CAD build for the part. Positions are in the model's coordinates, mm. Face numbers are marked on the shaded views. A direction names the side the tool comes from. Coordinates: 2 decimals unless noted, no trailing zeros. Write each loop counter-clockwise with the first axis right and the second up, starting at its lowest first coordinate (ties: lowest second). Pieces come first, ordered by that corner, then holes. Notation, with made-up numbers: (14, -13) - (49, -13) arc R26 ccw to (49, 1) - close; hole circle Ø1 at (46.25, -13). An arc over 180 degrees is marked (long way). Answer in a Markdown table with one row per item. Add a question column.
Q1. Band-saw the part on A-A (y = -3). List the corners of the cut face in (x, z).
Q2. Band-saw the part on C-C (z = -48). List the corners of the cut face in (x, y), and give its area (3 significant figures).
Q3. Pin check, flat tips, straight feed: pin 1 (2 mm diameter, centred on x = -77, z = -52.5, fed in from -Y); pin 2 (1.5 mm diameter, centred on x = -53, y = -4.5, fed in from +Z); pin 3 (8 mm diameter, centred on x = 34.5, y = -19, fed in from +Z). Stop position of each tip, or through.
Q4. Two-plate mould, pull along X, no slides. Class the marked faces 1, 2 and 3: +X half, -X half, draft (parallel to the pull), parting line (faces both ways), or undercut.
Q5. 3-axis set-ups, long thin cutter, end or side, ignore diameter. For the marked faces 4, 5, 6 and 7: which of +Z, -Z, +X, -X, +Y, -Y reach the whole face in a straight line?
Q6. Band-saw the part on B-B (x = 40). List the corners of the cut face in (y, z).
Q7. Band-saw the part on D-D (x = -35). List the corners of the cut face in (y, z).
Q8. Drill centre lines: line 1 along X through (y, z) = (-7, -26); line 2 along X through (y, z) = (-7, -30); line 3 along Z through (x, y) = (31.5, -21.5). Where is each one in solid material? Low to high. Write a range as from..to.
```python
from build123d import *

# Parameters (mm, degrees)
F0_W      = 160
F0_H      = 100
F1_DEPTH  = 20
F3_W      = 27
F3_H      = 100
F4_DEPTH  = 20
F5_DEPTH  = 20
F6_R      = 10
F7_DEPTH  = 30
F9_W      = 160
F9_H      = 27
F10_DEPTH = 20
F11_DEPTH = 20
F12_DEPTH = 20
F13_DEPTH = 20


with BuildPart() as f1:
    # F0 (on Front) → F1 (new body)
    with BuildSketch(Plane.XZ):
        Rectangle(F0_W, F0_H)
    extrude(amount=-F1_DEPTH)

    # F3 (on offset) → F4 (join)
    with BuildSketch(Plane.YZ.offset(-80)):
        with Locations((-13.5, 0)):
            Rectangle(F3_W, F3_H)
    extrude(amount=-F4_DEPTH)

    # F5 (add): faces of the model
    f5_faces = [f1.faces().sort_by_distance(p)[0] for p in [
        (-90, -27, 0),
        (-90, 0, 0),
    ]]
    extrude(f5_faces, amount=-F5_DEPTH, dir=(0, -1, 0))

    # F6 (on face) → F7 (join)
    with BuildSketch(Plane.XZ):
        with Locations((-40, -26.8495120108)):
            Circle(F6_R)
        with Locations((-40, 23.1504879892)):
            Circle(F6_R)
        with Locations((40, -26.8495120108)):
            Circle(F6_R)
        with Locations((40, 23.1504879892)):
            Circle(F6_R)
    extrude(amount=F7_DEPTH)



with BuildPart() as f10:
    # F9 (on offset) → F10 (new body)
    with BuildSketch(Plane.XY.offset(-50)):
        with Locations((0, -13.5)):
            Rectangle(F9_W, F9_H)
    extrude(amount=-F10_DEPTH)


with BuildPart() as f11:
    # F11 (new, through all): a face of the model
    f11_faces = [f10.part.faces().sort_by_distance(p)[0] for p in [
        (0, 0, -60),
    ]]
    extrude(f11_faces, amount=F11_DEPTH)


with BuildPart() as f12:
    # F12 (new, through all): a face of the model
    f12_faces = [f10.part.faces().sort_by_distance(p)[0] for p in [
        (-80, -13.5, -60),
    ]]
    extrude(f12_faces, amount=F12_DEPTH)


with BuildPart() as f1_1:
    add(f1.part)
    # F13 (add, through all): a face of the model
    f13_faces = [f11.part.faces().sort_by_distance(p)[0] for p in [
        (-80, 10, -60),
    ]]

    add(f10.part)  # F13 merges F10

    add(f11.part)  # F13 merges F11

    add(f12.part)  # F13 merges F12
    extrude(f13_faces, amount=F13_DEPTH)


solid = f1_1.part
```
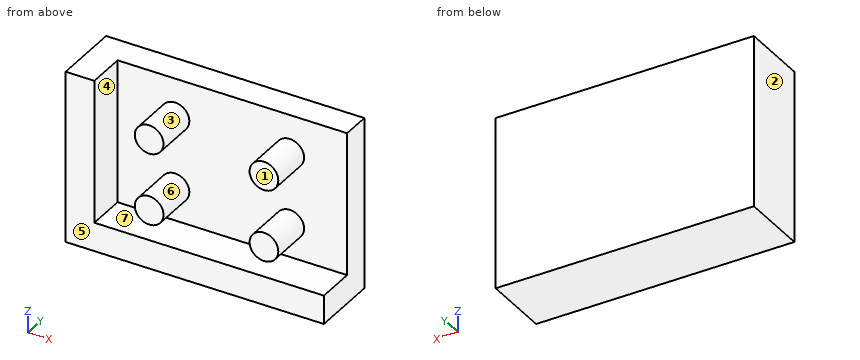
Checked values:
| question | item | result |
|---|---|---|
| 1 | outline | (-100, -70) - (80, -70) - (80, -50) - (-80, -50) - (-80, 50) - (-100, 50) - close; circle Ø20 at (-40, -26.85); circle Ø20 at (-40, 23.15); circle Ø20 at (40, -26.85); circle Ø20 at (40, 23.15) |
| 2 | outline | (-100, -27) - (-80, -27) - (-80, 0) - (80, 0) - (80, 20) - (-100, 20) - close |
| 2 | area | 4,140 mm² |
| 3 | pin 1 | stops at y = -27 |
| 3 | pin 2 | stops at z = -50 |
| 3 | pin 3 | stops at z = 33.04 |
| 4 | face 1 | draft |
| 4 | face 2 | -X half |
| 4 | face 3 | undercut |
| 5 | face 4 | +Z, -Y |
| 5 | face 5 | -Z, -X, -Y |
| 5 | face 6 | -Y |
| 5 | face 7 | +X, -Y |
| 6 | outline | (-30, -36.85) - (0, -36.85) - (0, -50) - (-27, -50) - (-27, -70) - (20, -70) - (20, 50) - (0, 50) - (0, 33.15) - (-30, 33.15) - (-30, 13.15) - (0, 13.15) - (0, -16.85) - (-30, -16.85) - close |
| 7 | outline | (-30, -35.51) - (0, -35.51) - (0, -50) - (-27, -50) - (-27, -70) - (20, -70) - (20, 50) - (0, 50) - (0, 31.81) - (-30, 31.81) - (-30, 14.49) - (0, 14.49) - (0, -18.19) - (-30, -18.19) - close |
| 8 | line 1 | x = -100..-80, -49.96..-30.04, 30.04..49.96 |
| 8 | line 2 | x = -100..-80, -49.49..-30.51, 30.51..49.49 |
| 8 | line 3 | z = -70..-50, -32.12..-21.58, 17.88..28.42 |
